```python
from build123d import *

# Parameters (mm, degrees)
CROQUIS1_W              = 30.5
CROQUIS1_H              = 20
CROQUIS1_R              = 1.5
SALIENTE_EXTRUIR1_DEPTH = 1.5
CROQUIS2_W              = 22
CROQUIS2_H              = 2.5
SALIENTE_EXTRUIR2_DEPTH = 2.75


with BuildPart() as part:
    # Croquis1 → Saliente-Extruir1 (new body)
    with BuildSketch(Plane(origin=(0, 0, 0), x_dir=(1, 0, 0), z_dir=(0, 1, 0))):
        Rectangle(CROQUIS1_W, CROQUIS1_H)
        with Locations(Location((-11.25, 7.37704918, 0), (0, 0, 270))):
            Circle(CROQUIS1_R, mode=Mode.SUBTRACT)
        with Locations(Location((11.25, -7.37704918, 0), (0, 0, 270))):
            Circle(CROQUIS1_R, mode=Mode.SUBTRACT)
    extrude(amount=SALIENTE_EXTRUIR1_DEPTH)

    # Croquis2 → Saliente-Extruir2 (add)
    with BuildSketch(Plane.XZ):
        with Locations((4.25, -8.25)):
            Rectangle(CROQUIS2_W, CROQUIS2_H)
    extrude(amount=SALIENTE_EXTRUIR2_DEPTH)


solid = part.part
```
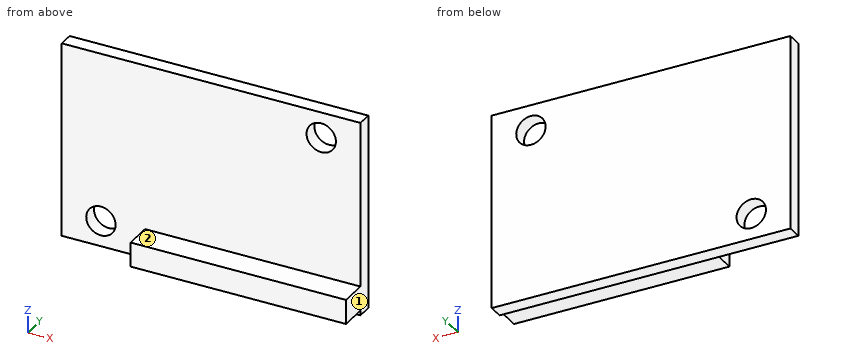
Here's how the part is built. I have some questions about the finished solid (model axes, mm). Face numbers are marked on the shaded views. A direction names the side the tool comes from. Coordinates: 2 decimals unless noted, no trailing zeros. Order: outer loops, then holes, each group sorted by start corner. A loop starts at its lowest first (then second) coordinate and runs counter-clockwise, first axis right, second up.
1) Which directions (+Z, -Z, +X, -X, +Y, -Y) give clear straight access to the entire face, cutting with the end or side of a thin tool? Please do the marked faces 1 and 2.
2) Imagine slicing it at D-D on x = -11.25. List the corners of the cut face in (y, z) for me.
3) I need wall thicknesses on line 1 (Y direction, x = 6, z = 3.25); line 2 (Z direction, x = 12, y = -1.15). Which ranges of each line are inside material? Lowest first, please.
4) Will these pins go through, and if not, where does the flat tip stop? pin 1 (1 mm diameter, centred on x = 4, y = -2.5, fed in from -Z); pin 2 (2.5 mm diameter, centred on x = -11.25, z = -7.38, fed in from +Y); pin 3 (0.8 mm diameter, centred on y = -1, z = -8, fed in from -X).
5) Imagine slicing it at A-A on x = 11.25. List the corners of the cut face in (y, z) for me, and give its area (3 significant figures).
6) Imagine slicing it at B-B on z = 6.25. List the corners of the cut face in (x, y) for me.
7) Imagine slicing it at C-C on y = 0.8. List the corners of the cut face in (x, z) for me, and give its area (3 significant figures).
Response values:
1. face 1: +Z, -Z, +X, +Y, -Y
1. face 2: +Z, +X, -X, -Y
2. outline: (0, -10) - (1.5, -10) - (1.5, -8.88) - (0, -8.88) - close; (0, -5.88) - (1.5, -5.88) - (1.5, 10) - (0, 10) - close
3. line 1: y = 0 to 1.5
3. line 2: z = -9.5 to -7
4. pin 1: stops at z = -9.5
4. pin 2: passes through
4. pin 3: stops at x = -6.75
5. outline: (-2.75, -9.5) - (0, -9.5) - (0, -10) - (1.5, -10) - (1.5, 5.88) - (0, 5.88) - (0, -7) - (-2.75, -7) - close; (0, 8.88) - (1.5, 8.88) - (1.5, 10) - (0, 10) - close
5. area: 32.4 mm2
6. outline: (-15.25, 0) - (10.26, 0) - (10.26, 1.5) - (-15.25, 1.5) - close; (12.24, 0) - (15.25, 0) - (15.25, 1.5) - (12.24, 1.5) - close
7. outline: (-15.25, -10) - (15.25, -10) - (15.25, 10) - (-15.25, 10) - close; hole circle Ø3 at (-11.25, -7.38); hole circle Ø3 at (11.25, 7.38)
7. area: 596 mm2
